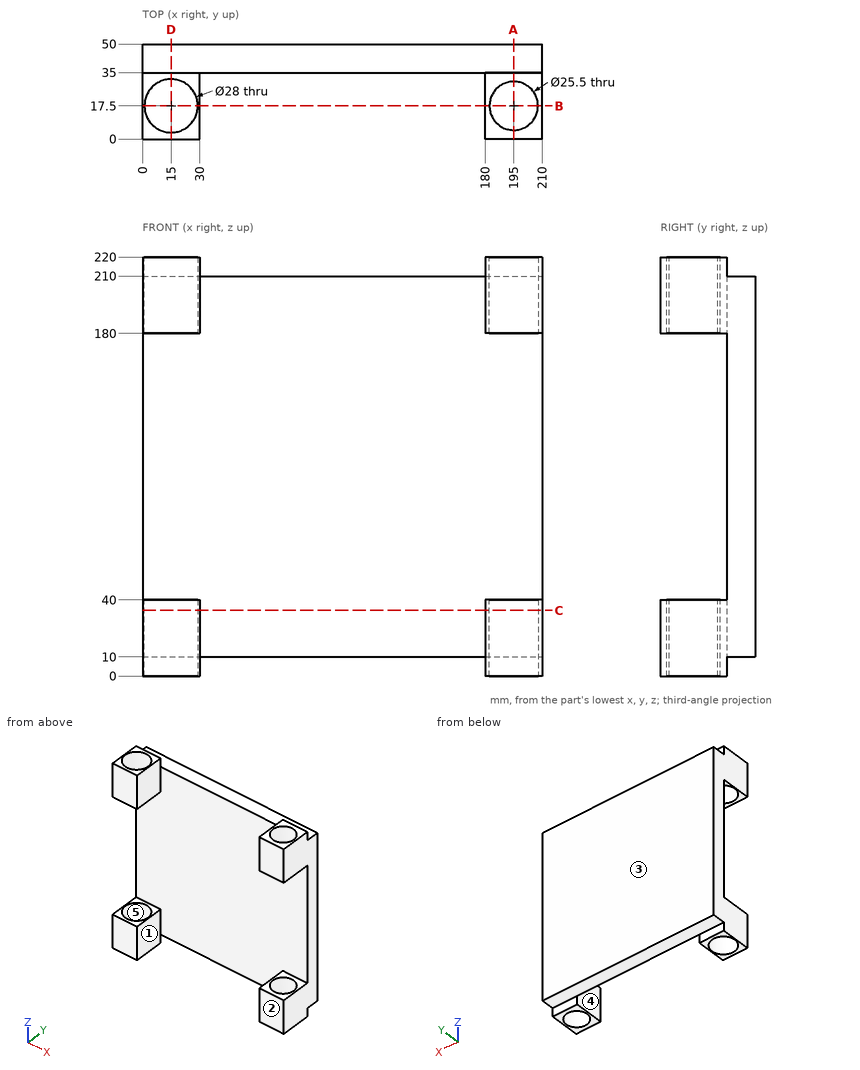
The drawing under review shows one solid part. Ordinate dimensions are in mm from its lowest x, y, z. A direction names the side the tool comes from. Give positions to 0.01 mm unless a question says otherwise; leave off trailing zeros. Write each loop counter-clockwise with the first axis right and the second up, starting at its lowest first coordinate (ties: lowest second). Pieces come first, ordered by that corner, then holes. Notation, with made-up numbers: (18, 36.25) - (72, 36.25) arc R36 cw to (72, 70.25) - close; hole circle Ø5 at (-32, 18.25). An arc over 180 degrees is marked (long way). Answer in a Markdown table with one row per item. Add a question column.
1. Insertion check: P1, Ø10, axis at x = 120, z = 56, coming from the -Y side; P2, Ø22.5, axis at x = 15, y = 17.5, coming from the -Z side; P3, Ø7.5, axis at x = 152, y = 41.5, coming from the -Z side; P4, Ø5, axis at x = 10, z = 216.5, coming from the +Y side. Each pin has a flat end and moves straight along its axis. Give the tip position at first contact, or say it passes through.
2. We need section D-D on x = 15. Write out the cut boundary in (y, z), then the cut area to 3 significant figures.
3. We need section B-B on y = 17.5. State how many separate pieces and enclosed holes the cut face has, then the cut area to 3 significant figures.
4. Draft analysis for pull direction Y (two halves, no side actions). For the marked faces 3, 4 and 5, state which applies: +Y half, -Y half, draft (parallel to the pull), parting line (faces both ways), or undercut.
5. Wall thickness on line 1 along X through (y, z) = (17, 205); line 2 along Y through (x, z) = (195, 203); line 3 along Y through (x, z) = (115.5, 177.5): over which ranges is each line inside the solid? List them lowest first. Write a range as [from, to].
6. Tool access review of the marked faces 1 and 2: name each direction out of +Z, -Z, +X, -X, +Y, -Y from which nothing blocks a thin tool from reaching the whole face with its end or side.
7. We need section C-C on z = 34.5. Write out the cut boundary in (x, y), then the cut area to 3 significant figures.
8. We need section A-A on x = 195. Write out the cut boundary in (y, z).
Ans:
| question | item | result |
|---|---|---|
| 1 | P1 | stops at y = 35 |
| 1 | P2 | passes through |
| 1 | P3 | stops at z = 10 |
| 1 | P4 | stops at y = 35 |
| 2 | outline | (0, 0) - (3.5, 0) - (3.5, 40) - (0, 40) - close; (0, 180) - (3.5, 180) - (3.5, 220) - (0, 220) - close; (31.5, 0) - (35, 0) - (35, 10) - (50, 10) - (50, 210) - (35, 210) - (35, 220) - (31.5, 220) - (31.5, 180) - (35, 180) - (35, 40) - (31.5, 40) - close |
| 2 | area | 3,560 mm^2 |
| 3 | separate pieces | 8 |
| 3 | enclosed holes | 0 |
| 3 | area | 520 mm^2 |
| 4 | face 3 | +Y half |
| 4 | face 4 | draft |
| 4 | face 5 | undercut |
| 5 | line 1 | x = [0, 1.01], [28.99, 30], [180, 182.26], [207.74, 210] |
| 5 | line 2 | y = [0, 4.75], [30.25, 50] |
| 5 | line 3 | y = [35, 50] |
| 6 | face 1 | +Z, -Z, -Y |
| 6 | face 2 | +Z, -Z, +X, -X, -Y |
| 7 | outline | (0, 0) - (30, 0) - (30, 35) - (180, 35) - (180, 0) - (210, 0) - (210, 50) - (0, 50) - close; hole circle Ø28 at (15, 17.5); hole circle Ø25.5 at (195, 17.5) |
| 7 | area | 4,120 mm^2 |
| 8 | outline | (0, 0) - (4.75, 0) - (4.75, 40) - (0, 40) - close; (0, 180) - (4.75, 180) - (4.75, 220) - (0, 220) - close; (30.25, 0) - (35, 0) - (35, 10) - (50, 10) - (50, 210) - (35, 210) - (35, 220) - (30.25, 220) - (30.25, 180) - (35, 180) - (35, 40) - (30.25, 40) - close |
